```python
from build123d import *

# Parameters (mm, degrees)
SKIZZE2_W                        = 120
SKIZZE2_H                        = 39.364160046
AUFSATZ_LINEAR_AUSTRAGEN1_DEPTH  = 30
SKIZZE24_R                       = 1.55
SCHNITT_LINEAR_AUSTRAGEN4_DEPTH  = 130.805766806
SKIZZE46_R                       = 2.85
SCHNITT_LINEAR_AUSTRAGEN15_DEPTH = 10
SCHNITT_LINEAR_START             = -5
SCHNITT_LINEAR_AUSTRAGEN25_DEPTH = 2.7
LINEARES_MUSTER1_COUNT           = 5
LINEARES_MUSTER1_PITCH           = 20
SPIEGELN2_COPY_1_SKETCH_R        = 2.85
SPIEGELN2_COPY_1_DEPTH           = 10
SPIEGELN2_COPY_2_SKETCH_R        = 2.85
SPIEGELN2_COPY_2_DEPTH           = 10
SPIEGELN2_COPY_3_SKETCH_R        = 2.85
SPIEGELN2_COPY_3_DEPTH           = 10
SPIEGELN2_COPY_4_SKETCH_R        = 2.85
SPIEGELN2_COPY_4_DEPTH           = 10
SPIEGELN2_START                  = -5
SPIEGELN2_COPY_5_DEPTH           = 2.7
SPIEGELN2_COPY_6_DEPTH           = 2.7
SPIEGELN2_COPY_7_DEPTH           = 2.7
SPIEGELN2_COPY_8_DEPTH           = 2.7
SKIZZE51_R                       = 1.55
SCHNITT_LINEAR_AUSTRAGEN26_DEPTH = 130.805766806
SKIZZE67_R                       = 0.425
SCHNITT_LINEAR_AUSTRAGEN30_DEPTH = 20
SKIZZE70_R                       = 0.5
SCHNITT_LINEAR_AUSTRAGEN37_DEPTH = 16
SKIZZE71_R                       = 2
SCHNITT_LINEAR_AUSTRAGEN38_DEPTH = 6
ABSPALTEN3_OUTLINE_W             = 120
ABSPALTEN3_OUTLINE_H             = 39.364160046
ABSPALTEN3_OUTLINE_R             = 1.55
ABSPALTEN3_DEPTH                 = 15


# Read off the part's stored shape, not the designer's step: Abspalten3
with BuildPart() as part:
    # Skizze2 → Aufsatz-Linear austragen1 (new body)
    with BuildSketch(Plane.XY):
        with Locations((60, 19.682080023)):
            Rectangle(SKIZZE2_W, SKIZZE2_H)
    extrude(amount=AUFSATZ_LINEAR_AUSTRAGEN1_DEPTH)

    # Skizze24 → Schnitt-Linear austragen4 (cut, through all)
    with BuildSketch(Plane.XY.offset(30)):
        with Locations((20, 31.364160046)):
            Circle(SKIZZE24_R)
        with Locations((40, 31.364160046)):
            Circle(SKIZZE24_R)
        with Locations((60, 31.364160046)):
            Circle(SKIZZE24_R)
        with Locations((80, 31.364160046)):
            Circle(SKIZZE24_R)
        with Locations((100, 31.364160046)):
            Circle(SKIZZE24_R)
    schnitt_linear_austragen4 = extrude(amount=-SCHNITT_LINEAR_AUSTRAGEN4_DEPTH, mode=Mode.SUBTRACT)

    # Skizze46 → Schnitt-Linear austragen15 (cut)
    with BuildSketch(Plane(origin=(0, 0, 0), x_dir=(-1, 0, 0), z_dir=(0, 0, -1))):
        with Locations((-100, 31.364160046)):
            Circle(SKIZZE46_R)
    schnitt_linear_austragen15 = extrude(amount=-SCHNITT_LINEAR_AUSTRAGEN15_DEPTH, mode=Mode.SUBTRACT)

    # Skizze50 → Schnitt-Linear austragen25 (cut)
    with BuildSketch(Plane.XY.offset(30).offset(SCHNITT_LINEAR_START)):
        Polygon((97.15, 33.009608314), (97.15, 39.364160046), (102.85, 39.364160046), (102.85, 33.009608314), (102.85, 29.718711779), (100, 28.073263512), (97.15, 29.718711779), align=None)
    schnitt_linear_austragen25 = extrude(amount=-SCHNITT_LINEAR_AUSTRAGEN25_DEPTH, mode=Mode.SUBTRACT)

    # Lineares Muster1: Schnitt-Linear austragen15, Schnitt-Linear austragen25 ×5
    with Locations(*[(-i * LINEARES_MUSTER1_PITCH, 0, 0) for i in range(1, LINEARES_MUSTER1_COUNT)]):
        add(schnitt_linear_austragen15, mode=Mode.SUBTRACT)
        add(schnitt_linear_austragen25, mode=Mode.SUBTRACT)

    # Spiegeln2: Schnitt-Linear austragen15, Schnitt-Linear austragen25 across plane
    add(schnitt_linear_austragen15.mirror(Plane.ZX.offset(19.764160046)), mode=Mode.SUBTRACT)
    add(schnitt_linear_austragen25.mirror(Plane.ZX.offset(19.764160046)), mode=Mode.SUBTRACT)

    # Spiegeln2 copy 1 sketch → Spiegeln2 copy 1 (cut)
    with BuildSketch(Plane(origin=(-20, 39.528320093, 0), x_dir=(-1, 0, 0), z_dir=(0, 0, -1))):
        with Locations((-100, -31.364160046)):
            Circle(SPIEGELN2_COPY_1_SKETCH_R)
    extrude(amount=-SPIEGELN2_COPY_1_DEPTH, mode=Mode.SUBTRACT)

    # Spiegeln2 copy 2 sketch → Spiegeln2 copy 2 (cut)
    with BuildSketch(Plane(origin=(-40, 39.528320093, 0), x_dir=(-1, 0, 0), z_dir=(0, 0, -1))):
        with Locations((-100, -31.364160046)):
            Circle(SPIEGELN2_COPY_2_SKETCH_R)
    extrude(amount=-SPIEGELN2_COPY_2_DEPTH, mode=Mode.SUBTRACT)

    # Spiegeln2 copy 3 sketch → Spiegeln2 copy 3 (cut)
    with BuildSketch(Plane(origin=(-60, 39.528320093, 0), x_dir=(-1, 0, 0), z_dir=(0, 0, -1))):
        with Locations((-100, -31.364160046)):
            Circle(SPIEGELN2_COPY_3_SKETCH_R)
    extrude(amount=-SPIEGELN2_COPY_3_DEPTH, mode=Mode.SUBTRACT)

    # Spiegeln2 copy 4 sketch → Spiegeln2 copy 4 (cut)
    with BuildSketch(Plane(origin=(-80, 39.528320093, 0), x_dir=(-1, 0, 0), z_dir=(0, 0, -1))):
        with Locations((-100, -31.364160046)):
            Circle(SPIEGELN2_COPY_4_SKETCH_R)
    extrude(amount=-SPIEGELN2_COPY_4_DEPTH, mode=Mode.SUBTRACT)

    # Spiegeln2 copy 5 sketch → Spiegeln2 copy 5 (cut)
    with BuildSketch(Plane(origin=(-20, 39.528320093, 30), x_dir=(1, 0, 0), z_dir=(0, 0, 1)).offset(SPIEGELN2_START)):
        Polygon((97.15, -33.009608314), (97.15, -39.364160046), (102.85, -39.364160046), (102.85, -33.009608314), (102.85, -29.718711779), (100, -28.073263512), (97.15, -29.718711779), align=None)
    extrude(amount=-SPIEGELN2_COPY_5_DEPTH, mode=Mode.SUBTRACT)

    # Spiegeln2 copy 6 sketch → Spiegeln2 copy 6 (cut)
    with BuildSketch(Plane(origin=(-40, 39.528320093, 30), x_dir=(1, 0, 0), z_dir=(0, 0, 1)).offset(SPIEGELN2_START)):
        Polygon((97.15, -33.009608314), (97.15, -39.364160046), (102.85, -39.364160046), (102.85, -33.009608314), (102.85, -29.718711779), (100, -28.073263512), (97.15, -29.718711779), align=None)
    extrude(amount=-SPIEGELN2_COPY_6_DEPTH, mode=Mode.SUBTRACT)

    # Spiegeln2 copy 7 sketch → Spiegeln2 copy 7 (cut)
    with BuildSketch(Plane(origin=(-60, 39.528320093, 30), x_dir=(1, 0, 0), z_dir=(0, 0, 1)).offset(SPIEGELN2_START)):
        Polygon((97.15, -33.009608314), (97.15, -39.364160046), (102.85, -39.364160046), (102.85, -33.009608314), (102.85, -29.718711779), (100, -28.073263512), (97.15, -29.718711779), align=None)
    extrude(amount=-SPIEGELN2_COPY_7_DEPTH, mode=Mode.SUBTRACT)

    # Spiegeln2 copy 8 sketch → Spiegeln2 copy 8 (cut)
    with BuildSketch(Plane(origin=(-80, 39.528320093, 30), x_dir=(1, 0, 0), z_dir=(0, 0, 1)).offset(SPIEGELN2_START)):
        Polygon((97.15, -33.009608314), (97.15, -39.364160046), (102.85, -39.364160046), (102.85, -33.009608314), (102.85, -29.718711779), (100, -28.073263512), (97.15, -29.718711779), align=None)
    extrude(amount=-SPIEGELN2_COPY_8_DEPTH, mode=Mode.SUBTRACT)

    # Spiegeln3: Schnitt-Linear austragen4 across plane
    add(schnitt_linear_austragen4.mirror(Plane.ZX.offset(19.764160046)), mode=Mode.SUBTRACT)

    # Skizze51 → Schnitt-Linear austragen26 (cut, through all)
    with BuildSketch(Plane.XY.offset(30)):
        with Locations((5, 34.364160046)):
            Circle(SKIZZE51_R)
        with Locations((115, 5)):
            Circle(SKIZZE51_R)
    extrude(amount=-SCHNITT_LINEAR_AUSTRAGEN26_DEPTH, mode=Mode.SUBTRACT)

    # Skizze66 → Schnitt-Rotation5 (revolve, cut)
    with BuildSketch(Plane.XY.offset(15), mode=Mode.PRIVATE) as schnitt_rotation5_sk:
        Polygon((110, 19.682080023), (110, 21.182080023), (10, 22.682080023), (10, 19.682080023), align=None)
        Polygon((105, 19.682080023), (105, 22.257192517), (15, 23.607192517), (15, 19.682080023), align=None)
    revolve(schnitt_rotation5_sk.sketch.rotate(Axis((10, 19.682080023, 15), (1, 0, 0)), 180), axis=Axis((10, 19.682080023, 15), (1, 0, 0)), mode=Mode.SUBTRACT)

    # Skizze67 → Schnitt-Linear austragen30 (cut)
    with BuildSketch(Plane(origin=(120, 0, 0), x_dir=(0, 0, -1), z_dir=(1, 0, 0))):
        with Locations((-17, 19.764160046)):
            Circle(SKIZZE67_R)
    schnitt_linear_austragen30 = extrude(amount=-SCHNITT_LINEAR_AUSTRAGEN30_DEPTH, mode=Mode.SUBTRACT)

    # Spiegeln7: Schnitt-Linear austragen30 across plane
    add(schnitt_linear_austragen30.mirror(Plane.XY.offset(15)), mode=Mode.SUBTRACT)

    # Skizze70 → Schnitt-Linear austragen37 (cut)
    with BuildSketch(Plane.ZY):
        with Locations((11.58373564, 19.764160046)):
            Circle(SKIZZE70_R)
    extrude(amount=-SCHNITT_LINEAR_AUSTRAGEN37_DEPTH, mode=Mode.SUBTRACT)

    # Skizze71 → Schnitt-Linear austragen38 (cut)
    with BuildSketch(Plane.ZY):
        with Locations((11.58373564, 19.764160046)):
            Circle(SKIZZE71_R)
    extrude(amount=-SCHNITT_LINEAR_AUSTRAGEN38_DEPTH, mode=Mode.SUBTRACT)

    # Abspalten3 outline → Abspalten3 (cut)
    with BuildSketch(Plane.XY):
        with Locations((60, 19.682080023)):
            Rectangle(ABSPALTEN3_OUTLINE_W, ABSPALTEN3_OUTLINE_H)
        with Locations((115, 5)):
            Circle(ABSPALTEN3_OUTLINE_R, mode=Mode.SUBTRACT)
        with Locations((5, 34.364160046)):
            Circle(ABSPALTEN3_OUTLINE_R, mode=Mode.SUBTRACT)
        with Locations((20, 8.164160046)):
            Circle(ABSPALTEN3_OUTLINE_R, mode=Mode.SUBTRACT)
        with Locations((40, 8.164160046)):
            Circle(ABSPALTEN3_OUTLINE_R, mode=Mode.SUBTRACT)
        with Locations((60, 8.164160046)):
            Circle(ABSPALTEN3_OUTLINE_R, mode=Mode.SUBTRACT)
        with Locations((80, 8.164160046)):
            Circle(ABSPALTEN3_OUTLINE_R, mode=Mode.SUBTRACT)
        with Locations((100, 8.164160046)):
            Circle(ABSPALTEN3_OUTLINE_R, mode=Mode.SUBTRACT)
        with Locations((20, 31.364160046)):
            Circle(ABSPALTEN3_OUTLINE_R, mode=Mode.SUBTRACT)
        with Locations((40, 31.364160046)):
            Circle(ABSPALTEN3_OUTLINE_R, mode=Mode.SUBTRACT)
        with Locations((60, 31.364160046)):
            Circle(ABSPALTEN3_OUTLINE_R, mode=Mode.SUBTRACT)
        with Locations((80, 31.364160046)):
            Circle(ABSPALTEN3_OUTLINE_R, mode=Mode.SUBTRACT)
        with Locations((100, 31.364160046)):
            Circle(ABSPALTEN3_OUTLINE_R, mode=Mode.SUBTRACT)
    extrude(amount=ABSPALTEN3_DEPTH, mode=Mode.SUBTRACT)


solid = part.part
```
Source: CAD feature listing. Evaluate the final solid. Frame: model axes, mm. A direction names the side the tool comes from. Coordinates: 2 decimals unless noted, no trailing zeros. Write each loop counter-clockwise with the first axis right and the second up, starting at its lowest first coordinate (ties: lowest second). Pieces come first, ordered by that corner, then holes. Notation, with made-up numbers: M 37.25,50 L 66.25,50 A9 ccw 66.25,55 Z; hole C -24.5,-16.5 d4. An arc over 180 degrees is marked long. Answer as a JSON object with one key per item and string values.
1. Cut plane C-C on x = 5. Output: boundary loops of the cut face in (y, z).
Evaluation:
{"outline": "M 0,15 L 32.81,15 L 32.81,30 L 0,30 Z; M 35.91,15 L 39.36,15 L 39.36,30 L 35.91,30 Z"}
2. Cut plane B-B on x = 115. Output: boundary loops of the cut face in (y, z) (3 decimals).
Evaluation:
{"outline": "M 0,15 L 3.45,15 L 3.45,30 L 0,30 Z; M 6.55,15 L 39.364,15 L 39.364,30 L 6.55,30 Z; hole C 19.764,17 d0.85"}
3. Ray query, L1, parallel to Y at x = 100, z = 19.75; L2, parallel to X at y = 38, z = 24.5; L3, parallel to Z at x = 39, y = 33. Return the intervals inside material, ascending.
Evaluation:
{"L1": "0 to 6.61, 9.71 to 29.81, 32.91 to 39.36", "L2": "0 to 17.15, 22.85 to 37.15, 42.85 to 57.15, 62.85 to 77.15, 82.85 to 97.15, 102.85 to 120", "L3": "15 to 22.3, 25 to 30"}
4. Cut plane A-A on y = 5. Output: boundary loops of the cut face in (x, z), plus the area to 3 significant figures.
Evaluation:
{"outline": "M 0,15 L 113.45,15 L 113.45,30 L 0,30 Z; M 116.55,15 L 120,15 L 120,30 L 116.55,30 Z; hole M 17.15,22.3 L 22.85,22.3 L 22.85,25 L 17.15,25 Z; hole M 37.15,22.3 L 42.85,22.3 L 42.85,25 L 37.15,25 Z; hole M 57.15,22.3 L 62.85,22.3 L 62.85,25 L 57.15,25 Z; hole M 77.15,22.3 L 82.85,22.3 L 82.85,25 L 77.15,25 Z; hole M 97.15,22.3 L 102.85,22.3 L 102.85,25 L 97.15,25 Z", "area": "1,680 mm^2"}
5. Access query for faces 1 (the flat face through (18.595, 28.884, 23.669)), 2 (the cylindrical face through (101.43, 30.77, 27.54)), 3 (the flat face through (40, 0.164, 24)). Directions: +Z, -Z, +X, -X, +Y, -Y. A direction counts if a zero-diameter tool reaches every point of the face in a straight line with its end or side. Return the directions, or none.
Evaluation:
{"face 1": "+Y", "face 2": "+Z, -Z", "face 3": "none"}
6. Draft query along Z for faces 4 (the flat face through (17.15, 5, 24)), 5 (the flat face through (120, 19, 22)), 6 (the flat face through (59, 20, 30)). Return one class per face: released by +Z, released by -Z, zero draft, split by the parting line, or undercut.
Evaluation:
{"face 4": "undercut", "face 5": "zero draft", "face 6": "released by +Z"}
7. Cut plane D-D on z = 28.75. State how many separate pieces and enclosed holes the cut face has, plus the area to 3 significant figures.
Evaluation:
{"separate pieces": "1", "enclosed holes": "12", "area": "4,630 mm^2"}
